Answer from the drawing. Dimensions are ordinates in mm from the lowest x, y and z of the part. A direction names the side the tool comes from. Round coordinates to 2 decimals unless told otherwise and drop trailing zeros. Order: outer loops, then holes, each group sorted by start corner. A loop starts at its lowest first (then second) coordinate and runs counter-clockwise, first axis right, second up. Notation, with made-up numbers: M 81,89.25 L 123,89.25 A29 ccw 123,119.25 Z; hole C 45,77.5 d9. An arc over 180 degrees is marked long. Write item = value, one per line. Start each with the question number.
(1) Which of the six approach directions +Z, -Z, +X, -X, +Y, -Y give full straight-line access (tool end or side, diameter ignored) to the marked faces 1, 2 and 3?
(2) A cutting plane is placed at A-A, the plane y = 9. Determine the outline of the cut face in (x, z).
(3) For a pull along X with two mould halves and no side action, classify the marked faces 4, 5 and 6 as released by +X, released by -X, zero draft, split by the parting line, or undercut.
(4) A cutting plane is placed at C-C, the plane z = 27.5. Determine the outline of the cut face in (x, y).
(5) Straight lines are drawn through the part: probe 1 along Y at (x, z) = (36, 9); probe 2 along Y at (x, z) = (36.5, 34.5); probe 3 along Y at (x, z) = (9.5, 38). For each, find the intervals that lie inside material, in ascending order. Write a range as from..to.
(6) Each of these flat-tipped pins is pushed along its axis until it touches: pin 1 (5 mm diameter, centred on x = 19, y = 23, fed in from +Z); pin 2 (6 mm diameter, centred on x = 18.5, z = 25.5, fed in from +Y); pin 3 (16.5 mm diameter, centred on x = 33, z = 26, fed in from +Y). Where does it stop, or does it pass through?
(7) A cutting plane is placed at D-D, the plane z = 8. Determine the outline of the cut face in (x, y).
(8) A cutting plane is placed at B-B, the plane x = 39. Determine the outline of the cut face in (y, z).
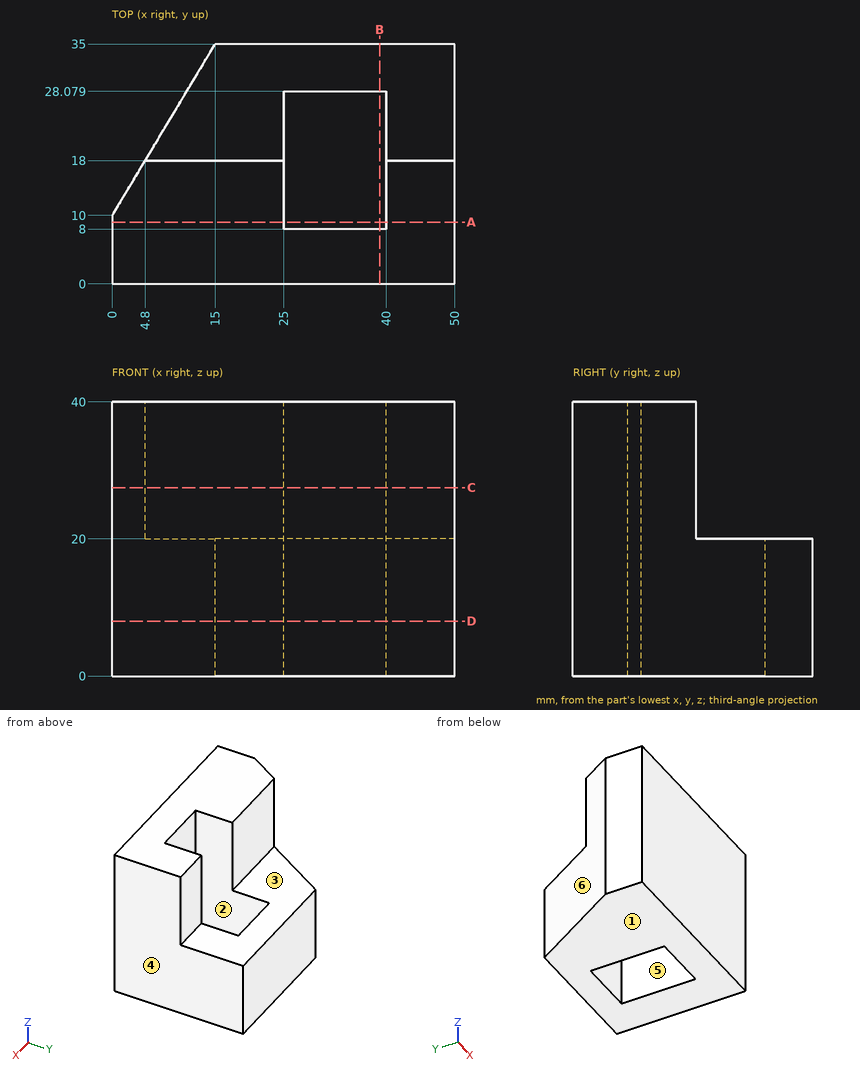
Reported:
q1.face_1 = -Z, +X, -X, +Y, -Y
q1.face_2 = +Z, -Z
q1.face_3 = +Z, +X, -X, +Y
q2.outline = M 0,0 L 25,0 L 25,40 L 0,40 Z; M 40,0 L 50,0 L 50,40 L 40,40 Z
q3.face_4 = released by +X
q3.face_5 = undercut
q3.face_6 = released by -X
q4.outline = M 0,0 L 50,0 L 50,18 L 40,18 L 40,8 L 25,8 L 25,18 L 4.8,18 L 0,10 Z
q5.probe_1 = 0..8, 28.08..35
q5.probe_2 = 0..8
q5.probe_3 = 0..18
q6.pin_1 = 20
q6.pin_2 = 18
q6.pin_3 = 35
q7.outline = M 0,0 L 50,0 L 50,35 L 15,35 L 0,10 Z; hole M 25,8 L 40,8 L 40,28.08 L 25,28.08 Z
q8.outline = M 0,0 L 8,0 L 8,40 L 0,40 Z; M 28.08,0 L 35,0 L 35,20 L 28.08,20 Z
